Part model, mm, in its own coordinate system. Coordinates: 2 decimals unless noted, no trailing zeros. Write each loop counter-clockwise with the first axis right and the second up, starting at its lowest first coordinate (ties: lowest second). Pieces come first, ordered by that corner, then holes. Notation, with made-up numbers: (82, 55.5) - (94, 55.5) arc R19 cw to (94, 72.5) - close; hole circle Ø5 at (-2, 49.5). An arc over 180 degrees is marked (long way). Use a Markdown table: item, result.
```python
from build123d import *

# Parameters (mm, degrees)
SKETCH1_W           = 62
SKETCH1_H           = 62
SKETCH1_R           = 2
BOSS_EXTRUDE1_DEPTH = 4
SKETCH2_R           = 18
CUT_EXTRUDE1_DEPTH  = 10
FILLET1_R           = 5


with BuildPart() as part:
    # Sketch1 → Boss-Extrude1 (new body)
    with BuildSketch(Plane(origin=(0, 0, 0), x_dir=(1, 0, 0), z_dir=(0, 1, 0))):
        Rectangle(SKETCH1_W, SKETCH1_H)
        with Locations((25.5, 25.5)):
            Circle(SKETCH1_R, mode=Mode.SUBTRACT)
        with Locations((-25.5, 25.5)):
            Circle(SKETCH1_R, mode=Mode.SUBTRACT)
        with Locations((25.5, -25.5)):
            Circle(SKETCH1_R, mode=Mode.SUBTRACT)
        with Locations((-25.5, -25.5)):
            Circle(SKETCH1_R, mode=Mode.SUBTRACT)
    extrude(amount=BOSS_EXTRUDE1_DEPTH)

    # Sketch2 → Cut-Extrude1 (cut)
    with BuildSketch(Plane(origin=(0, 4, 0), x_dir=(1, 0, 0), z_dir=(0, 1, 0))):
        Circle(SKETCH2_R)
    extrude(amount=-CUT_EXTRUDE1_DEPTH, mode=Mode.SUBTRACT)

    # Fillet1
    fillet1_edges = [part.edges().sort_by_distance(p)[0] for p in [
        (-31, 2, 31),
        (-31, 2, -31),
        (31, 2, -31),
        (31, 2, 31),
    ]]
    fillet(fillet1_edges, radius=FILLET1_R)


solid = part.part
```
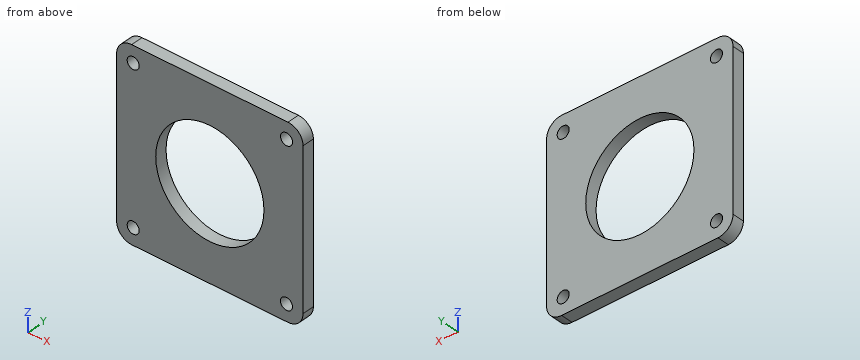
Item 1: Band-saw the part on B-B, the plane z = 0. Give the cut face in (x, y).
From the geometry:
| item | result |
|---|---|
| outline | (-31, 0) - (-18, 0) - (-18, 4) - (-31, 4) - close; (18, 0) - (31, 0) - (31, 4) - (18, 4) - close |
Item 2: Band-saw the part on A-A, the plane x = 0. Give the cut face in (y, z).
From the geometry:
| item | result |
|---|---|
| outline | (0, -31) - (4, -31) - (4, -18) - (0, -18) - close; (0, 18) - (4, 18) - (4, 31) - (0, 31) - close |
Item 3: Drill centre lines: probe 1 along X at (y, z) = (2, 25.5); probe 2 along X at (y, z) = (2.65, 0). Where is each one in solid material? Low to high.
From the geometry:
| item | result |
|---|---|
| probe 1 | -31 to -27.5, -23.5 to 23.5, 27.5 to 31 |
| probe 2 | -31 to -18, 18 to 31 |
